The model under review builds one solid part; all positions refer to its coordinate system, in mm. Coordinates: 2 decimals unless noted, no trailing zeros. Write each loop counter-clockwise with the first axis right and the second up, starting at its lowest first coordinate (ties: lowest second). Pieces come first, ordered by that corner, then holes.
1) For line 1 (Y direction, x = -0.3, z = 1.4); line 2 (X direction, y = 5, z = 0.95); line 3 (Z direction, x = -0.55, y = 9), list the stretches that pass through material, from the lowest coordinate up.
2) Add section C-C, the plane y = 10.5. State the section outline as (x, z) points (1 decimal).
3) Add section B-B, the plane x = -0.95. State the section outline as (y, z) points.
4) Add section A-A, the plane z = 0.45. State the section outline as (x, y) points.
from build123d import *

# Parameters (mm, degrees)
SKETCH1_R           = 1.5875
BOSS_EXTRUDE1_DEPTH = 16.51
SKETCH3_R           = 1.903344521
SKETCH3_R_2         = 1.27
CUT_EXTRUDE2_DEPTH  = 0.254


with BuildPart() as part:
    # Sketch1 → Boss-Extrude1 (new body)
    with BuildSketch(Plane(origin=(0, 0, 0), x_dir=(1, 0, 0), z_dir=(0, 1, 0))):
        with Locations(Location((0, 0, 0), (0, 0, 270))):
            Circle(SKETCH1_R)
    extrude(amount=BOSS_EXTRUDE1_DEPTH)

    # Sketch3 → Cut-Extrude2 (cut)
    with BuildSketch(Plane(origin=(0, 1.27, 0), x_dir=(-1, 0, 0), z_dir=(0, -1, 0))):
        Circle(SKETCH3_R)
        with Locations(Location((0, 0, 0), (0, 0, 90))):
            Circle(SKETCH3_R_2, mode=Mode.SUBTRACT)
    cut_extrude2 = extrude(amount=-CUT_EXTRUDE2_DEPTH, mode=Mode.SUBTRACT)

    # Mirror2: Cut-Extrude2 across plane
    add(cut_extrude2.mirror(Plane(origin=(0, 8.255, 0), x_dir=(0, 0, 1), z_dir=(0, -1, 0))), mode=Mode.SUBTRACT)


solid = part.part
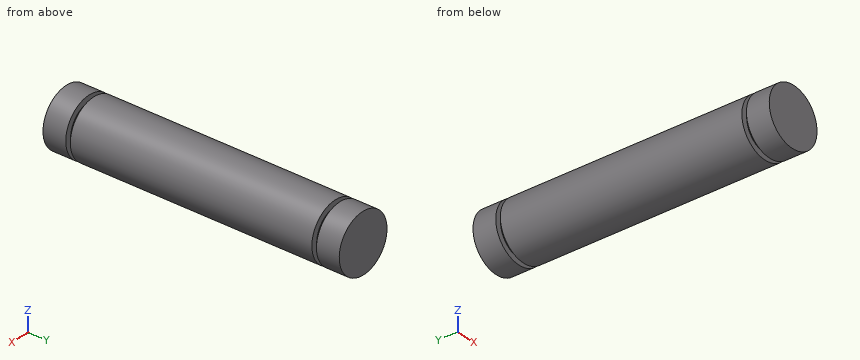
Geometry results:
1. line 1: y = 0 to 1.27, 1.52 to 14.99, 15.24 to 16.51
1. line 2: x = -1.27 to 1.27
1. line 3: z = -1.49 to 1.49
2. outline: circle Ø3.2 at (0, 0)
3. outline: (0, -1.27) - (1.27, -1.27) - (1.27, -0.84) - (1.52, -0.84) - (1.52, -1.27) - (14.99, -1.27) - (14.99, -0.84) - (15.24, -0.84) - (15.24, -1.27) - (16.51, -1.27) - (16.51, 1.27) - (15.24, 1.27) - (15.24, 0.84) - (14.99, 0.84) - (14.99, 1.27) - (1.52, 1.27) - (1.52, 0.84) - (1.27, 0.84) - (1.27, 1.27) - (0, 1.27) - close
4. outline: (-1.52, 0) - (1.52, 0) - (1.52, 1.27) - (1.19, 1.27) - (1.19, 1.52) - (1.52, 1.52) - (1.52, 14.99) - (1.19, 14.99) - (1.19, 15.24) - (1.52, 15.24) - (1.52, 16.51) - (-1.52, 16.51) - (-1.52, 15.24) - (-1.19, 15.24) - (-1.19, 14.99) - (-1.52, 14.99) - (-1.52, 1.52) - (-1.19, 1.52) - (-1.19, 1.27) - (-1.52, 1.27) - close
